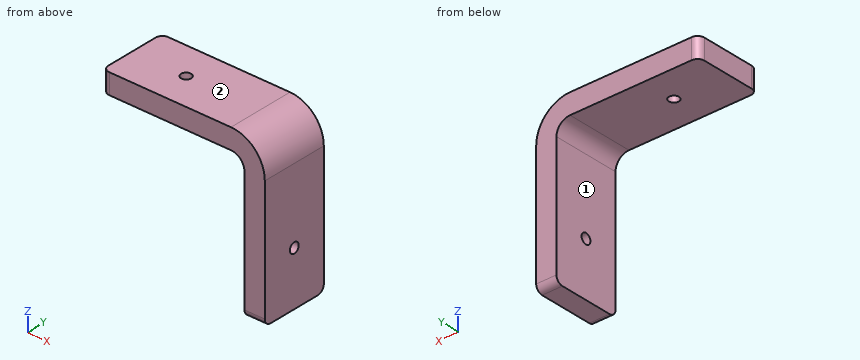
from build123d import *

# Parameters (mm, degrees)
F1_DEPTH = 31.75
F2_R     = 2.3876
F3_DEPTH = 25.4
F4_R     = 2.3876
F5_DEPTH = 25.4
F6_R     = 15.875
F7_R     = 6.35
F8_R     = 3.175


with BuildPart() as f1:
    # F0 (on Front) → F1 (new body)
    with BuildSketch(Plane.XZ):
        Polygon((66.675, 66.675), (66.675, 0), (76.2, 0), (76.2, 76.2), (0, 76.2), (0, 66.675), align=None)
    extrude(amount=F1_DEPTH)

    # F2 (on face) → F3 (cut)
    with BuildSketch(Plane.YZ.offset(76.2)):
        with Locations((-15.875, 25.4)):
            Circle(F2_R)
    extrude(amount=-F3_DEPTH, mode=Mode.SUBTRACT)

    # F4 (on face) → F5 (cut)
    with BuildSketch(Plane.XY.offset(76.2)):
        with Locations((25.4, -15.875)):
            Circle(F4_R)
    extrude(amount=-F5_DEPTH, mode=Mode.SUBTRACT)

    # F6
    f6_edges = [f1.edges().sort_by_distance(p)[0] for p in [
        (76.2, -15.875, 76.2),
    ]]
    fillet(f6_edges, radius=F6_R)

    # F7
    f7_edges = [f1.edges().sort_by_distance(p)[0] for p in [
        (66.675, -15.875, 66.675),
    ]]
    fillet(f7_edges, radius=F7_R)

    # F8
    f8_edges = [f1.edges().sort_by_distance(p)[0] for p in [
        (0, 0, 71.4375),
        (0, -31.75, 71.4375),
        (71.4375, 0, 0),
        (71.4375, -31.75, 0),
    ]]
    fillet(f8_edges, radius=F8_R)


solid = f1.part
Build history of the part. All positions in model axes, mm. Face numbers are marked on the shaded views. A direction names the side the tool comes from. Give positions to 0.01 mm unless a question says otherwise; leave off trailing zeros. Loops run counter-clockwise (first coordinate to the right, second up) from the corner with the lowest first, then second, coordinate; pieces in that order, holes last. Notation, with made-up numbers: (-39.5, -35.75) -> (4.5, -35.75) arc R26 cw to (4.5, -12.75) -> close; hole circle Ø3 at (-5, 23.25). An arc over 180 degrees is marked (long way). Answer in a Markdown table with one row per item.
Item 1: Tool access for the marked faces 1 and 2: list every direction of +Z, -Z, +X, -X, +Y, -Y with a clear straight run to the whole face (end or side of a thin tool).
Findings below:
| item | result |
|---|---|
| face 1 | -Z, -X, +Y, -Y |
| face 2 | +Z, +X, -X, +Y, -Y |
Item 2: Slice it at C-C on y = -11. Write the cut outline in (x, z) (3 decimals).
Findings below:
| item | result |
|---|---|
| outline | (0, 66.675) -> (60.325, 66.675) arc R6.35 cw to (66.675, 60.325) -> (66.675, 0) -> (76.2, 0) -> (76.2, 60.325) arc R15.875 ccw to (60.325, 76.2) -> (0, 76.2) -> close |
Item 3: Slice it at A-A on z = 25.4. Write the cut outline in (x, y) (3 decimals), plus the area to 3 significant figures.
Findings below:
| item | result |
|---|---|
| outline | (66.675, -31.75) -> (76.2, -31.75) -> (76.2, -18.263) -> (66.675, -18.263) -> close; (66.675, -13.487) -> (76.2, -13.487) -> (76.2, 0) -> (66.675, 0) -> close |
| area | 257 mm² |
Item 4: Slice it at B-B on x = 25.4. Write the cut outline in (y, z) (3 decimals).
Findings below:
| item | result |
|---|---|
| outline | (-31.75, 66.675) -> (-18.263, 66.675) -> (-18.263, 76.2) -> (-31.75, 76.2) -> close; (-13.487, 66.675) -> (0, 66.675) -> (0, 76.2) -> (-13.487, 76.2) -> close |
Item 5: Flat gauge pins, fed straight in: P1, Ø4, axis at y = -26.5, z = 37, coming from the -X side (3 decimals); P2, Ø3, axis at x = 25.4, y = -15.875, coming from the +Z side; P3, Ø1, axis at x = 34, y = -25.5, coming from the -Z side (3 decimals); P4, Ø6, axis at y = -25, z = 59, coming from the -X side. Where does each tip first touch, or does it go through?
Findings below:
| item | result |
|---|---|
| P1 | stops at x = 66.675 |
| P2 | passes through |
| P3 | stops at z = 66.675 |
| P4 | stops at x = 66.45 |
Item 6: Slice it at D-D on z = 62. Write the cut outline in (x, y).
Findings below:
| item | result |
|---|---|
| outline | (66.45, -31.75) -> (76.11, -31.75) -> (76.11, 0) -> (66.45, 0) -> close |
Item 7: Probe line 1 along Y through (x, z) = (25.4, 72.25); line 2 along Z through (x, y) = (45, -29) (3 decimals). List the from-to ranges inside material, lowest first. Write a range as [from, to].
Findings below:
| item | result |
|---|---|
| line 1 | y = [-31.75, -18.26], [-13.49, 0] |
| line 2 | z = [66.675, 76.2] |
